Check sheet for the drawn part. Datum: minimum x, y, z corner. Units: mm. Coordinates: 2 decimals unless noted, no trailing zeros. Loops run counter-clockwise (first coordinate to the right, second up) from the corner with the lowest first, then second, coordinate; pieces in that order, holes last. Notation, with made-up numbers: (-5.5, 29) - (40.5, 29) arc R26 cw to (40.5, 65) - close; hole circle Ø8 at (64, 9). An arc over 180 degrees is marked (long way). Answer as a JSON object with one key per item and string values. Group by question number.
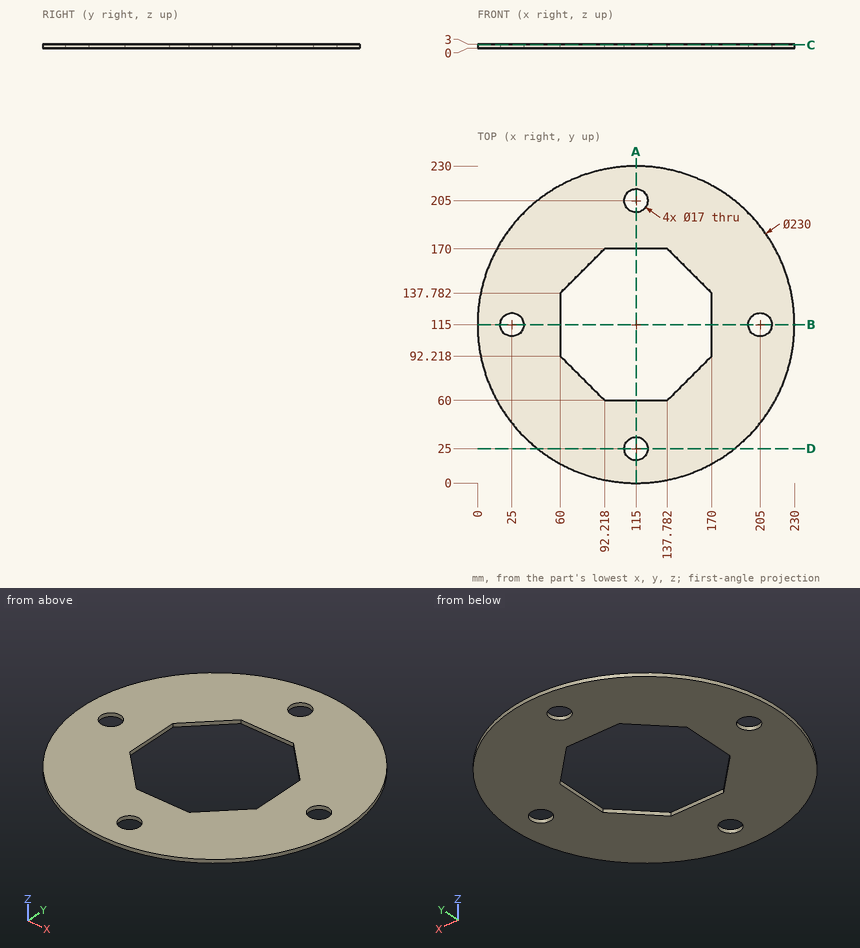
1. Sectioned sample at D-D on y = 25. Record the cut outline in (x, z).
2. Gauge pin test, flat ends, axial feed: pin 1 (1.5 mm diameter, centred on x = 137, z = 2, fed in from +Y); pin 2 (1.5 mm diameter, centred on y = 52.5, z = 0.5, fed in from +X) (1 decimal); pin 3 (0.9 mm diameter, centred on y = 124.5, z = 1, fed in from +X); pin 4 (3 mm diameter, centred on x = 30.5, y = 170.5, fed in from -Z). Record the tip position at first contact, or that the pin passes through.
3. Sectioned sample at A-A on x = 115. Record the cut outline in (y, z).
4. Material ranges on line 1 (Y direction, x = 115, z = 1.95); line 2 (Y direction, x = 119.5, z = 2.65); line 3 (Y direction, x = 88, z = 0.8) (1 decimal), recorded low to high.
5. Sectioned sample at C-C on z = 2.3. Record the cut outline in (x, y), plus the area to 3 significant figures.
Answers follow:
{
 "1": {"outline": "(43.41, 0) - (106.5, 0) - (106.5, 3) - (43.41, 3) - close; (123.5, 0) - (186.59, 0) - (186.59, 3) - (123.5, 3) - close"},
 "2": {"pin 1": "stops at y = 228.02", "pin 2": "stops at x = 212", "pin 3": "stops at x = 229.64", "pin 4": "stops at z = 0"},
 "3": {"outline": "(0, 0) - (16.5, 0) - (16.5, 3) - (0, 3) - close; (33.5, 0) - (60, 0) - (60, 3) - (33.5, 3) - close; (170, 0) - (196.5, 0) - (196.5, 3) - (170, 3) - close; (213.5, 0) - (230, 0) - (230, 3) - (213.5, 3) - close"},
 "4": {"line 1": "y = 0 to 16.5, 33.5 to 60, 170 to 196.5, 213.5 to 230", "line 2": "y = 0.09 to 17.79, 32.21 to 60, 170 to 197.79, 212.21 to 229.91", "line 3": "y = 3.2 to 64.2, 165.8 to 226.8"},
 "5": {"outline": "circle Ø230 at (115, 115); hole circle Ø17 at (25, 115); hole (60, 92.22) - (92.22, 60) - (137.78, 60) - (170, 92.22) - (170, 137.78) - (137.78, 170) - (92.22, 170) - (60, 137.78) - close; hole circle Ø17 at (115, 25); hole circle Ø17 at (115, 205); hole circle Ø17 at (205, 115)", "area": "30,600 mm^2"}
}
